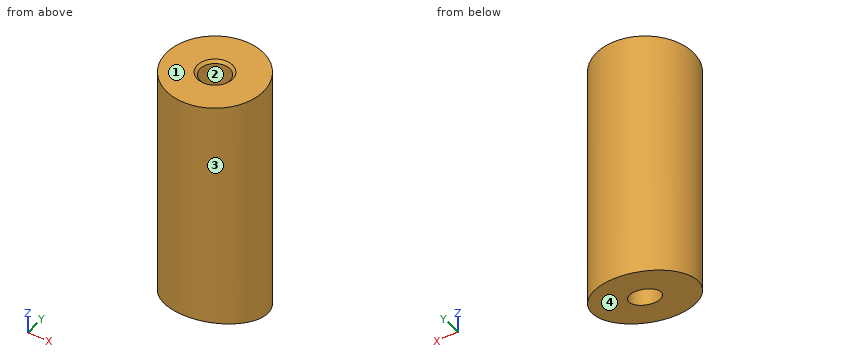
```python
from build123d import *

# Parameters (mm, degrees)
SKIZZE1_W                       = 58.664904562
SKIZZE1_H                       = 11.08559322
SCHNITT_LINEAR_AUSTRAGEN1_DEPTH = 13
M8_GEWINDEBOHRUNG1_D            = 6.8
M8_GEWINDEBOHRUNG1_DEPTH        = 22.25
M8_GEWINDEBOHRUNG1_CSINK_D      = 8.05
M8_GEWINDEBOHRUNG1_CSINK_ANGLE  = 90
M8_GEWINDEBOHRUNG1_TIP          = 2.042926105
M8_GEWINDEBOHRUNG2_D            = 6.8
M8_GEWINDEBOHRUNG2_DEPTH        = 22.25
M8_GEWINDEBOHRUNG2_CSINK_D      = 8.05
M8_GEWINDEBOHRUNG2_CSINK_ANGLE  = 90
M8_GEWINDEBOHRUNG2_TIP          = 2.042926105


with BuildPart() as part:
    # Skizze1 → Rotation1 (revolve)
    with BuildSketch(Plane(origin=(0, 0, 0), x_dir=(0, 0, -1), z_dir=(1, 0, 0)), mode=Mode.PRIVATE) as rotation1_sk:
        with Locations((29.332452281, 5.54279661)):
            Rectangle(SKIZZE1_W, SKIZZE1_H)
    revolve(rotation1_sk.sketch.rotate(Axis((0, 0, 0), (0, 0, -1)), 90), axis=Axis((0, 0, 0), (0, 0, -1)))  # turned: the seam where the file's is

    # Skizze2 → Schnitt-Linear austragen1 (cut, symmetric)
    with BuildSketch(Plane(origin=(0, 0, 0), x_dir=(0, 0, -1), z_dir=(1, 0, 0))):
        Polygon((58.664904562, 11.08559322), (52.72415306, -11.08559322), (58.664904562, -11.08559322), align=None)
    extrude(amount=SCHNITT_LINEAR_AUSTRAGEN1_DEPTH, both=True, mode=Mode.SUBTRACT)

    # M8 Gewindebohrung1
    with Locations(Plane.XY):
        with Locations((0, 0)):
            CounterSinkHole(M8_GEWINDEBOHRUNG1_D / 2, M8_GEWINDEBOHRUNG1_CSINK_D / 2, depth=M8_GEWINDEBOHRUNG1_DEPTH, counter_sink_angle=M8_GEWINDEBOHRUNG1_CSINK_ANGLE)
            with Locations((0, 0, -(M8_GEWINDEBOHRUNG1_DEPTH + M8_GEWINDEBOHRUNG1_TIP / 2))):  # 118° drill point
                Cone(0, M8_GEWINDEBOHRUNG1_D / 2, M8_GEWINDEBOHRUNG1_TIP, mode=Mode.SUBTRACT)

    # M8 Gewindebohrung2
    with Locations(Plane(origin=(0, 0, -58.664904562), x_dir=(1, 0, 0), z_dir=(0, 0, -1))):
        with Locations((0, 0)):
            CounterSinkHole(M8_GEWINDEBOHRUNG2_D / 2, M8_GEWINDEBOHRUNG2_CSINK_D / 2, depth=M8_GEWINDEBOHRUNG2_DEPTH, counter_sink_angle=M8_GEWINDEBOHRUNG2_CSINK_ANGLE)
            with Locations((0, 0, -(M8_GEWINDEBOHRUNG2_DEPTH + M8_GEWINDEBOHRUNG2_TIP / 2))):  # 118° drill point
                Cone(0, M8_GEWINDEBOHRUNG2_D / 2, M8_GEWINDEBOHRUNG2_TIP, mode=Mode.SUBTRACT)


solid = part.part
```
Can you work these out from the model? Positions are in its coordinate system, mm. Face numbers are marked on the shaded views. Coordinates: 2 decimals unless noted, no trailing zeros. Loops run counter-clockwise (first coordinate to the right, second up) from the corner with the lowest first, then second, coordinate; pieces in that order, holes last.
1) Imagine slicing it at A-A on z = -50. List the corners of the cut face in (x, y) for me.
2) Imagine slicing it at D-D on x = -7.75. List the corners of the cut face in (y, z) for me.
3) Thinking about a two-plate mould opening in Y: for the marked faces 1, 2, 3 and 4, which applies, pulls with the +Y half, pulls with the -Y half, needs draft (parallel to the pull), parting line crosses it, or undercut?
4) Imagine slicing it at C-C on y = 5.5. List the corners of the cut face in (x, z) for me.
5) Imagine slicing it at B-B on z = -25. List the corners of the cut face in (x, y) for me, plus the area to 3 significant figures.
6) I need wall thicknesses on probe 1 along Y at (x, z) = (0, -46.25); probe 2 along X at (y, z) = (0.25, -5.5); probe 3 along Z at (x, y) = (4.75, 0.25). Which ranges of each line are inside material? Lowest first, please.
7) For pin 1 (1 mm diameter, centred on y = 5, z = -24.5, fed in from -X); pin 2 (1 mm diameter, centred on x = 4, y = 2.5, fed in from +Z); pin 3 (8 mm diameter, centred on x = 0, y = 0, fed in from -Z); pin 4 (6 mm diameter, centred on y = 5, z = -9.5, fed in from -X), each with a flat end and sliding along its axis, tell me the tip position at first contact or that it passes through.
Completed:
1. outline: circle Ø22.17 at (0, 0); hole circle Ø6.8 at (0, 0)
2. outline: (-7.93, -53.57) - (7.93, -57.82) - (7.93, 0) - (-7.93, 0) - close
3. face 1: needs draft
3. face 2: undercut
3. face 3: parting line crosses it
3. face 4: pulls with the -Y half
4. outline: (-9.62, -57.17) - (9.62, -57.17) - (9.62, 0) - (-9.62, 0) - close
5. outline: circle Ø22.17 at (0, 0)
5. area: 386 mm2
6. probe 1: y = -11.09 to -3.4, 3.4 to 11.09
6. probe 2: x = -11.08 to -3.39, 3.39 to 11.08
6. probe 3: z = -55.76 to 0
7. pin 1: stops at x = -10.13
7. pin 2: stops at z = 0
7. pin 3: stops at z = -56.77
7. pin 4: stops at x = -10.9
